Geometry: final body of the model. Coordinates: model frame, mm. A direction names the side the tool comes from. Round coordinates to 2 decimals unless told otherwise and drop trailing zeros. Order: outer loops, then holes, each group sorted by start corner. A loop starts at its lowest first (then second) coordinate and runs counter-clockwise, first axis right, second up. Notation, with made-up numbers: M -25.5,24.5 L -5.5,24.5 A17 ccw -5.5,40.5 Z; hole C 57,81 d10. An arc over 180 degrees is marked long. Put each result on its own line as item: value. Start each with the question number.
1) Draft query along Z for faces 1 (the cylindrical face through (33.72, 59.22, -66.18)), 2 (the cylindrical face through (13.35, 55.765, -63.479)), 3 (the cylindrical face through (-39.965, 44.543, -12.759)). Return one class per face: pulls with the +Z half, pulls with the -Z half, needs draft (parallel to the pull), parting line crosses it, or undercut.
2) First-contact query: P1, Ø2.5, axis at x = 22, y = 58.69, coming from the +Z side; P2, Ø5, axis at x = 37.5, y = 30, coming from the -Z side; P3, Ø4, axis at x = -7.5, z = -67.5, coming from the -Y side; P4, Ø5, axis at x = 30, y = 58.69, coming from the +Z side. Flat tips, straight axial feed; report the tip coordinate or a pass-through.
3) Section B-B, the plane y = 8.5. Return loops of the section in (x, z).
4) Section A-A, the plane x = -22. Return loops of the section in (y, z).
5) Section D-D, the plane x = 39.5. Return loops of the section in (y, z).
6) Access query for faces 4 (the flat face through (23, 57, -65)), 5 (the cylindrical face through (39.96, 41.82, -21.34)), 6 (the flat face through (-42.51, 45.3, -24.6)). Directions: +Z, -Z, +X, -X, +Y, -Y. A direction counts if a zero-diameter tool reaches every point of the face in a straight line with its end or side. Return the directions, or none.
7) Material intervals for probe 1 along X at (y, z) = (62, -67); probe 2 along Y at (x, z) = (-14, -64.15); probe 3 along Y at (x, z) = (-22, -67), sorted ascending. Write a range as [from, to].
8) Section C-C, the plane z = -12.5. Return loops of the section in (x, y), then the cut area to 3 significant figures.
from build123d import *

# Parameters (mm, degrees)
SKETCH_1_W               = 120
SKETCH_1_H               = 8
EXTRUDE_1_DEPTH          = 5
SKETCH_2_W               = 5.019384612
SKETCH_2_H               = 8
PATTERN_LINEAR_2_COUNT   = 2
PATTERN_LINEAR_2_PITCH   = 80
EXTRUDE_3_DEPTH          = 6
EXTRUDE_3_DEPTH_BACK     = 2
SKETCH_5_W               = 85.019384612
SKETCH_5_H               = 9.428556335
SKETCH_6_R               = 1.52
CUT_EXTRUDE_1_DEPTH      = 18
PATTERN_LINEAR_3_COUNT   = 3
PATTERN_LINEAR_3_PITCH   = 8
MIRROR_1_COPY_1_SKETCH_R = 1.52
MIRROR_1_COPY_1_DEPTH    = 18
MIRROR_1_COPY_2_SKETCH_R = 1.52
MIRROR_1_COPY_2_DEPTH    = 18
SKETCH_7_R               = 1.52
CUT_EXTRUDE_2_DEPTH      = 15
SKETCH_8_W               = 136.689726825
SKETCH_8_H               = 40.838827277
CUT_EXTRUDE_3_DEPTH      = 8
SKETCH_10_R              = 3
CUT_EXTRUDE_5_DEPTH      = 3
FILLET_1_R               = 1.5
FILLET_2_R               = 1.5


with BuildPart() as part:
    # 草图1 → 凸台-拉伸1 (new body)
    with BuildSketch(Plane(origin=(0, 0, 0), x_dir=(1, 0, 0), z_dir=(0, 1, 0))):
        Rectangle(SKETCH_1_W, SKETCH_1_H)
    extrude(amount=EXTRUDE_1_DEPTH)

    # 扫描2: sweep along a curve in space
    with BuildLine() as sweep_2_path:
        ThreePointArc((-40, 5, 0), (-40, 46.186296303, -20.238339114), (-40, 60, -64))
    # 草图2 → 扫描2 (sweep)
    with BuildSketch(Plane(origin=(0, 5, 0), x_dir=(1, 0, 0), z_dir=(0, 1, 0))):
        with Locations((-40, 0)):
            Rectangle(SKETCH_2_W, SKETCH_2_H)
    sweep_2 = sweep(path=sweep_2_path.line)

    # 阵列(线性)2: 扫描2 ×2
    with Locations(*[(i * PATTERN_LINEAR_2_PITCH, 0, 0) for i in range(1, PATTERN_LINEAR_2_COUNT)]):
        add(sweep_2)

    # 草图5 → 凸台-拉伸3 (add, two sides: drawn at the far end of the back side and taken through both)
    with BuildSketch(Plane(origin=(0, 0, -64), x_dir=(-1, 0, 0), z_dir=(0, 0, -1)).offset(-EXTRUDE_3_DEPTH_BACK)):
        with Locations((0, 59.281524703)):
            Rectangle(SKETCH_5_W, SKETCH_5_H)
    extrude(amount=EXTRUDE_3_DEPTH + EXTRUDE_3_DEPTH_BACK)

    # 草图6 → 切除-拉伸1 (cut)
    with BuildSketch(Plane(origin=(0, 0, -70), x_dir=(-1, 0, 0), z_dir=(0, 0, -1))):
        with Locations((30, 58.693516137)):
            Circle(SKETCH_6_R)
    cut_extrude_1 = extrude(amount=-CUT_EXTRUDE_1_DEPTH, mode=Mode.SUBTRACT)

    # 阵列(线性)3: 切除-拉伸1 ×3
    with Locations(*[(i * PATTERN_LINEAR_3_PITCH, 0, 0) for i in range(1, PATTERN_LINEAR_3_COUNT)]):
        add(cut_extrude_1, mode=Mode.SUBTRACT)

    # 镜向1: 切除-拉伸1 across plane
    add(cut_extrude_1.mirror(Plane(origin=(0, 0, 0), x_dir=(0, 0, 1), z_dir=(1, 0, 0))), mode=Mode.SUBTRACT)

    # 镜向1 copy 1 sketch → 镜向1 copy 1 (cut)
    with BuildSketch(Plane(origin=(-8, 0, -70), x_dir=(1, 0, 0), z_dir=(0, 0, -1))):
        with Locations((30, -58.693516137)):
            Circle(MIRROR_1_COPY_1_SKETCH_R)
    extrude(amount=-MIRROR_1_COPY_1_DEPTH, mode=Mode.SUBTRACT)

    # 镜向1 copy 2 sketch → 镜向1 copy 2 (cut)
    with BuildSketch(Plane(origin=(-16, 0, -70), x_dir=(1, 0, 0), z_dir=(0, 0, -1))):
        with Locations((30, -58.693516137)):
            Circle(MIRROR_1_COPY_2_SKETCH_R)
    extrude(amount=-MIRROR_1_COPY_2_DEPTH, mode=Mode.SUBTRACT)

    # 草图7 → 切除-拉伸2 (cut)
    with BuildSketch(Plane(origin=(0, 54.567246535, 0), x_dir=(-1, 0, 0), z_dir=(0, -1, 0))):
        with Locations(Location((0, 67, 0), (0, 0, 90))):
            Circle(SKETCH_7_R)
        with Locations(Location((35, 67, 0), (0, 0, 90))):
            Circle(SKETCH_7_R)
        with Locations(Location((-35, 67, 0), (0, 0, 270))):
            Circle(SKETCH_7_R)
    extrude(amount=-CUT_EXTRUDE_2_DEPTH, mode=Mode.SUBTRACT)

    # 草图8 → 切除-拉伸3 (cut)
    with BuildSketch(Plane(origin=(0, 63.99580287, 0), x_dir=(1, 0, 0), z_dir=(0, 1, 0))):
        with Locations((2.188010226, 52.474472022)):
            Rectangle(SKETCH_8_W, SKETCH_8_H)
    extrude(amount=CUT_EXTRUDE_3_DEPTH, mode=Mode.SUBTRACT)

    # 草图10 → 切除-拉伸5 (cut)
    with BuildSketch(Plane.XY.offset(-62)):
        with Locations((30, 58.693516137)):
            Circle(SKETCH_10_R)
        with Locations((22, 58.693516137)):
            Circle(SKETCH_10_R)
        with Locations((14, 58.693516137)):
            Circle(SKETCH_10_R)
        with Locations(Location((-30, 58.693516137, 0), (0, 0, 180))):
            Circle(SKETCH_10_R)
        with Locations(Location((-22, 58.693516137, 0), (0, 0, 180))):
            Circle(SKETCH_10_R)
        with Locations(Location((-14, 58.693516137, 0), (0, 0, 180))):
            Circle(SKETCH_10_R)
    extrude(amount=-CUT_EXTRUDE_5_DEPTH, mode=Mode.SUBTRACT)

    # 圆角1
    fillet_1_edges = [part.edges().sort_by_distance(p)[0] for p in [
        (40, 56.159889336, -62),
    ]]
    fillet(fillet_1_edges, radius=FILLET_1_R)

    # 圆角2
    fillet_2_edges = [part.edges().sort_by_distance(p)[0] for p in [
        (-40, 56.159889336, -62),
    ]]
    fillet(fillet_2_edges, radius=FILLET_2_R)


solid = part.part
Result sheet:
1. face 1: undercut
1. face 2: needs draft
1. face 3: pulls with the +Z half
2. P1: passes through
2. P2: stops at z = -13.32
2. P3: stops at y = 54.57
2. P4: stops at z = -65
3. outline: M -42.51,-4.31 L -37.49,-4.31 L -37.49,3.73 L -42.51,3.73 Z; M 37.49,-4.31 L 42.51,-4.31 L 42.51,3.73 L 37.49,3.73 Z
4. outline: M 0,-4 L 5,-4 L 5,4 L 0,4 Z; M 54.57,-70 L 57.17,-70 L 57.17,-65 L 55.69,-65 L 55.69,-62 L 54.57,-62 Z; M 60.21,-70 L 64,-70 L 64,-62 L 61.69,-62 L 61.69,-65 L 60.21,-65 Z
5. outline: M 0,-4 L 5,-4 A54.35 cw 56.24,-60.56 A1.5 cw 54.74,-62 L 54.57,-62 L 54.57,-70 L 64,-70 L 64,-52.35 A62.34 ccw 5,4 L 0,4 Z
6. face 4: +Z
6. face 5: +X, -X, -Y
6. face 6: +Z, -Z, -X, +Y
7. probe 1: x = [-42.51, -36.52], [-33.48, -1.52], [1.52, 33.48], [36.52, 42.51]
7. probe 2: y = [54.57, 55.69], [61.69, 64]
7. probe 3: y = [54.57, 57.17], [60.21, 64]
8. outline: M -42.51,31.25 L -37.49,31.25 L -37.49,44.27 L -42.51,44.27 Z; M 37.49,31.25 L 42.51,31.25 L 42.51,44.27 L 37.49,44.27 Z
8. area: 131 mm2
